For this review, take the finished solid that the model builds, in its own axes (mm). A direction names the side the tool comes from. Round coordinates to 2 decimals unless told otherwise and drop trailing zeros. Order: outer loops, then holes, each group sorted by start corner. A loop starts at its lowest first (then second) coordinate and runs counter-clockwise, first axis right, second up.
```python
from build123d import *

# Parameters (mm, degrees)
CORTAR_EXTRUIR1_DEPTH = 2
CHAFL_N1_SIZE         = 0.5
REDONDEO1_R           = 0.5


with BuildPart() as part:
    # Croquis1 → Revolución1 (revolve)
    with BuildSketch(Plane.XY):
        Polygon((0, 0), (2.75, 0), (2.75, -3), (1.5, -3), (1.5, -15), (0, -15), align=None)
    revolve(axis=Axis((0, 0, 0), (0, -1, 0)))

    # Croquis2 → Cortar-Extruir1 (cut)
    with BuildSketch(Plane(origin=(0, 0, 0), x_dir=(1, 0, 0), z_dir=(0, 1, 0))):
        Polygon((1.25, 0.721687836), (0, 1.443375673), (-1.25, 0.721687836), (-1.25, -0.721687836), (0, -1.443375673), (1.25, -0.721687836), align=None)
    extrude(amount=-CORTAR_EXTRUIR1_DEPTH, mode=Mode.SUBTRACT)

    # Chaflán1
    chafl_n1_edges = [part.edges().sort_by_distance(p)[0] for p in [
        (-1.5, -15, 0),
    ]]
    chamfer(chafl_n1_edges, length=CHAFL_N1_SIZE)

    # Redondeo1
    redondeo1_edges = [part.edges().sort_by_distance(p)[0] for p in [
        (-2.75, 0, 0),
    ]]
    fillet(redondeo1_edges, radius=REDONDEO1_R)


solid = part.part
```
Q1. Take a section at A-A, the plane y = -1.25. State the section outline as (x, z) points.
Q2. Tool access review of faces 1 (the face through (0.63, -0.99, -1.08)), 2 (the face through (1.2, -3, -1.2)), 3 (the face through (-0.596, -1.768, -2.685)): name each direction out of +Z, -Z, +X, -X, +Y, -Y from which nothing blocks a thin tool from reaching the whole face with its end or side.
Q3. Wall thickness on line 1 (Y direction, x = -0.45, z = 0.3); line 2 (Y direction, x = -2.1, z = -0.7); line 3 (X direction, y = -13.25, z = 0.1): over which ranges is each line inside the solid? List them lowest first.
Q4. Take a section at B-B, the plane z = 0. State the section outline as (x, y) points, plus the area to 3 significant figures.
Q5. Clearance check with flat-ended pins moving along their axes: pin 1 (3 mm diameter, centred on y = -8.5, z = 2, fed in from -X); pin 2 (1 mm diameter, centred on x = -0.5, z = -2, fed in from -Y). State where each tip first meets the part, or that it passes through.
Q6. Take a section at C-C, the plane y = -10.5. State the section outline as (x, z) points, plus the area to 3 significant figures.
Q7. Mouldability with a two-part tool opening along Z and no side actions: class faces 4 (the face through (-1.5, -8.83, 0.07)), 5 (the face through (1.25, -1, 0)), 6 (the face through (-1.5, 0, 0)) as +Z half, -Z half, draft (parallel to the pull), parting line (faces both ways), or undercut.
Working result:
1. outline: circle Ø5.5 at (0, 0); hole (-1.25, -0.72) - (0, -1.44) - (1.25, -0.72) - (1.25, 0.72) - (0, 1.44) - (-1.25, 0.72) - close
2. face 1: +Y
2. face 2: -Y
2. face 3: +Y, -Y
3. line 1: y = -15 to -2
3. line 2: y = -3 to 0
3. line 3: x = -1.5 to 1.5
4. outline: (-2.75, -3) - (-1.5, -3) - (-1.5, -14.5) - (-1, -15) - (1, -15) - (1.5, -14.5) - (1.5, -3) - (2.75, -3) - (2.75, -0.5) arc R0.5 ccw to (2.25, 0) - (1.25, 0) - (1.25, -2) - (-1.25, -2) - (-1.25, 0) - (-2.25, 0) arc R0.5 ccw to (-2.75, -0.5) - close
4. area: 47.1 mm2
5. pin 1: stops at x = -1.41
5. pin 2: stops at y = -3
6. outline: circle Ø3 at (0, 0)
6. area: 7.07 mm2
7. face 4: parting line
7. face 5: undercut
7. face 6: draft
